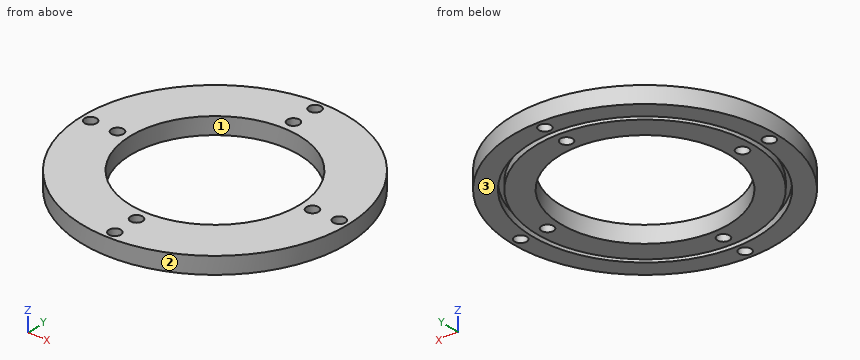
```python
from build123d import *

# Parameters (mm, degrees)
SKETCH1_R           = 45
SKETCH1_R_2         = 35
SKETCH1_R_3         = 2.5
BOSS_EXTRUDE1_DEPTH = 7
SKETCH2_R           = 55
SKETCH2_R_2         = 47.047288935
BOSS_EXTRUDE3_DEPTH = 7
BOSS_EXTRUDE4_START = -4
SKETCH3_R           = 47.047288935
SKETCH3_R_2         = 45
BOSS_EXTRUDE4_DEPTH = 4
SKETCH4_R           = 2.5
CUT_EXTRUDE1_DEPTH  = 79.096094653


with BuildPart() as part:
    # Sketch1 → Boss-Extrude1 (new body)
    with BuildSketch(Plane.XY):
        with Locations(Location((0, 0, 0), (0, 0, 180))):
            Circle(SKETCH1_R)
        with Locations(Location((0, 0, 0), (0, 0, 180))):
            Circle(SKETCH1_R_2, mode=Mode.SUBTRACT)
        with Locations(Location((0, 40, 0), (0, 0, 180))):
            Circle(SKETCH1_R_3, mode=Mode.SUBTRACT)
        with Locations(Location((40, 0, 0), (0, 0, 180))):
            Circle(SKETCH1_R_3, mode=Mode.SUBTRACT)
        with Locations(Location((0, -40, 0), (0, 0, 180))):
            Circle(SKETCH1_R_3, mode=Mode.SUBTRACT)
        with Locations(Location((-40, 0, 0), (0, 0, 180))):
            Circle(SKETCH1_R_3, mode=Mode.SUBTRACT)
    extrude(amount=BOSS_EXTRUDE1_DEPTH)



with BuildPart() as body_2:
    # Sketch2 → Boss-Extrude3 (new body)
    with BuildSketch(Plane.XY.offset(7)):
        Circle(SKETCH2_R)
        Circle(SKETCH2_R_2, mode=Mode.SUBTRACT)
    extrude(amount=-BOSS_EXTRUDE3_DEPTH)


with BuildPart() as part_1:
    add(part.part)

    add(body_2.part)  # Boss-Extrude4 merges body 2
    # Sketch3 → Boss-Extrude4 (add)
    with BuildSketch(Plane.XY.offset(7).offset(BOSS_EXTRUDE4_START)):
        Circle(SKETCH3_R)
        with Locations(Location((0, 0, 0), (0, 0, 180))):
            Circle(SKETCH3_R_2, mode=Mode.SUBTRACT)
    extrude(amount=BOSS_EXTRUDE4_DEPTH)

    # Sketch4 → Cut-Extrude1 (cut, through all)
    with BuildSketch(Plane(origin=(0, 0, 0), x_dir=(-1, 0, 0), z_dir=(0, 0, -1))):
        with Locations((0, -51.023644468)):
            Circle(SKETCH4_R)
        with Locations((-51.023644468, 0)):
            Circle(SKETCH4_R)
        with Locations((0, 51.023644468)):
            Circle(SKETCH4_R)
        with Locations((51.023644468, 0)):
            Circle(SKETCH4_R)
    extrude(amount=-CUT_EXTRUDE1_DEPTH, mode=Mode.SUBTRACT)


solid = part_1.part
```
Geometry check sheet. Reference: the model listing, model coordinates, mm. Face numbers are marked on the shaded views. Coordinates: 2 decimals unless noted, no trailing zeros. Write each loop counter-clockwise with the first axis right and the second up, starting at its lowest first coordinate (ties: lowest second). Pieces come first, ordered by that corner, then holes. Notation, with made-up numbers: (63.5, -38.5) -> (79.5, -38.5) arc R22 cw to (79.5, -15.5) -> close; hole circle Ø7 at (-12, 61). An arc over 180 degrees is marked (long way). Use CSV: the item, a comma, the result in double quotes. Start each with the question number.
Item 1: Cross-section at A-A, the plane z = 1.25. State how many separate pieces and enclosed holes the cut face has, plus the area to 3 significant figures.
Item 2: Cross-section at B-B, the plane x = 7. Record the cut outline in (y, z).
Item 3: Cross-section at C-C, the plane y = -17. Record the cut outline in (x, z), plus the area to 3 significant figures.
Item 4: Mould release check, pull along Y, two halves, no side actions. Record for the marked faces 1, 2 and 3: released by +Y, released by -Y, zero draft, split by the parting line, or undercut.
Item 5: Depth check by flat-ended pin: pin 1 Ø3 at (x, z) = (20.5, 6) entering from +Y; pin 2 Ø4 at (x, z) = (-13, 1.5) entering from -Y. Enter the tip coordinate at first touch or a pass-through.
Item 6: Thickness scan on line 1 (Y direction, x = 0, z = 3.25); line 2 (Y direction, x = 20, z = 1.25); line 3 (Y direction, x = 9.5, z = 1). Record the ranges inside material, lowest first.
Answers:
1,separate pieces,"2"
1,enclosed holes,"10"
1,area,"4,910 mm^2"
2,outline,"(-54.55, 0) -> (-46.52, 0) -> (-46.52, 3) -> (-44.45, 3) -> (-44.45, 0) -> (-34.29, 0) -> (-34.29, 7) -> (-54.55, 7) -> close; (34.29, 0) -> (44.45, 0) -> (44.45, 3) -> (46.52, 3) -> (46.52, 0) -> (54.55, 0) -> (54.55, 7) -> (34.29, 7) -> close"
3,outline,"(-52.31, 0) -> (-43.87, 0) -> (-43.87, 3) -> (-41.67, 3) -> (-41.67, 0) -> (-30.59, 0) -> (-30.59, 7) -> (-52.31, 7) -> close; (30.59, 0) -> (41.67, 0) -> (41.67, 3) -> (43.87, 3) -> (43.87, 0) -> (52.31, 0) -> (52.31, 7) -> (30.59, 7) -> close"
3,area,"291 mm^2"
4,face 1,"undercut"
4,face 2,"split by the parting line"
4,face 3,"zero draft"
5,pin 1,"y = 51.61"
5,pin 2,"y = -53.89"
6,line 1,"-55 to -53.52, -48.52 to -42.5, -37.5 to -35, 35 to 37.5, 42.5 to 48.52, 53.52 to 55"
6,line 2,"-51.23 to -42.58, -40.31 to -28.72, 28.72 to 40.31, 42.58 to 51.23"
6,line 3,"-54.17 to -46.08, -43.99 to -33.69, 33.69 to 43.99, 46.08 to 54.17"
